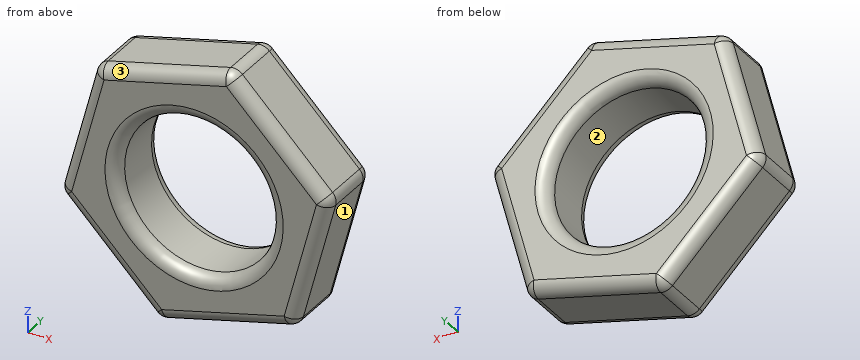
```python
from build123d import *

# Parameters (mm, degrees)
SKETCH1_R           = 4
BOSS_EXTRUDE1_DEPTH = 3.556
FILLET1_R           = 0.635
FILLET2_R           = 0.635


with BuildPart() as part:
    # Sketch1 → Boss-Extrude1 (new body)
    with BuildSketch(Plane(origin=(0, 0, 0), x_dir=(1, 0, 0), z_dir=(0, 1, 0))):
        Polygon((5.205006366, 5.164420787), (-1.870016414, 7.089878133), (-7.07502278, 1.925457346), (-5.205006366, -5.164420787), (1.870016414, -7.089878133), (7.07502278, -1.925457346), align=None)
        with Locations(Location((0, 0, 0), (0, 0, 270))):
            Circle(SKETCH1_R, mode=Mode.SUBTRACT)
    extrude(amount=BOSS_EXTRUDE1_DEPTH)

    # Fillet1
    fillet1_edges = [part.edges().sort_by_distance(p)[0] for p in [
        (0, 0, -4),
        (0, 3.556, -4),
    ]]
    fillet(fillet1_edges, radius=FILLET1_R)

    # Fillet2
    fillet2_edges = [part.edges().sort_by_distance(p)[0] for p in [
        (-4.472519597, 3.556, -4.50766774),
        (7.07502278, 1.778, 1.925457346),
        (1.870016414, 1.778, 7.089878133),
        (-5.205006366, 1.778, 5.164420787),
        (-7.07502278, 1.778, -1.925457346),
        (-1.870016414, 1.778, -7.089878133),
        (5.205006366, 1.778, -5.164420787),
        (-6.140014573, 3.556, 1.61948172),
        (-1.667494976, 3.556, 6.12714946),
        (4.472519597, 3.556, 4.50766774),
        (6.140014573, 3.556, -1.61948172),
        (4.472519597, 0, 4.50766774),
        (-1.667494976, 0, 6.12714946),
        (-6.140014573, 0, 1.61948172),
        (1.667494976, 3.556, -6.12714946),
        (-4.472519597, 0, -4.50766774),
        (1.667494976, 0, -6.12714946),
        (6.140014573, 0, -1.61948172),
    ]]
    fillet(fillet2_edges, radius=FILLET2_R)


solid = part.part
```
Geometry check sheet. Reference: the model listing, model coordinates, mm. Face numbers are marked on the shaded views. Give positions to 0.01 mm unless a question says otherwise; leave off trailing zeros. Loops run counter-clockwise (first coordinate to the right, second up) from the corner with the lowest first, then second, coordinate; pieces in that order, holes last. Notation, with made-up numbers: (10, -6) - (21, -6) arc R9 cw to (21, 7) - close; hole circle Ø2 at (-25, 82). An arc over 180 degrees is marked (long way). Use CSV: the item, a comma, the result in double quotes. Start each with the question number.
Q1. Go/stop test with flat-tipped pins: pin 1 Ø1.5 at (y, z) = (1.5, 1) entering from -X; pin 2 Ø1 at (y, z) = (2, -1) entering from +X; pin 3 Ø2 at (x, y) = (4.5, 1) entering from +Z. Record where each tip stops, or that it passes through.
Q2. Section check A-A, the plane y = 1.4. Record the cut outline in (x, z) (1 decimal).
Q3. Release check for a two-part mould opening along X. For the marked faces 1, 2 and 3 record: +X half, -X half, draft (parallel to the pull), parting line (faces both ways), or undercut.
Q4. Scan lines: probe 1 along X at (y, z) = (1.65, 0); probe 2 along X at (y, z) = (1.3, 0.25); probe 3 along Z at (x, y) = (2.5, 1.75). Record each from-to range of solid material in increasing order. Write a range as from..to.
Findings below:
1,pin 1,"stops at x = -6.5"
1,pin 2,"stops at x = 6.44"
1,pin 3,"stops at z = 5.47"
2,outline,"(-7, -1.6) arc R0.6 ccw to (-6.8, -2.2) - (-2.1, -6.8) arc R0.6 ccw to (-1.5, -7) - (4.9, -5.3) arc R0.6 ccw to (5.3, -4.8) - (7, 1.6) arc R0.6 ccw to (6.8, 2.2) - (2.1, 6.8) arc R0.6 ccw to (1.5, 7) - (-4.9, 5.3) arc R0.6 ccw to (-5.3, 4.8) - close; hole circle Ø8 at (0, 0)"
3,face 1,"+X half"
3,face 2,"undercut"
3,face 3,"-X half"
4,probe 1,"x = -6.57..-4, 4..6.57"
4,probe 2,"x = -6.5..-3.99, 3.99..6.63"
4,probe 3,"z = -5.9..-3.12, 3.12..6.46"
